Input: part model. Units: mm. Frame: model coordinates. Face numbers are marked on the shaded views. A direction names the side the tool comes from. Give positions to 0.01 mm unless a question says otherwise; leave off trailing zeros. Write each loop counter-clockwise with the first axis right and the second up, starting at its lowest first coordinate (ties: lowest second). Pieces come first, ordered by that corner, then holes.
```python
from build123d import *

# Parameters (mm, degrees)
SKETCH2_R           = 1.5
BOSS_EXTRUDE1_DEPTH = 2.5
SKETCH3_W           = 5.5
SKETCH3_H           = 2
BOSS_EXTRUDE2_DEPTH = 9
SKETCH4_W           = 5.5
SKETCH4_H           = 16.5
BOSS_EXTRUDE3_DEPTH = 2
SKETCH5_W           = 5.5
SKETCH5_H           = 2
BOSS_EXTRUDE4_DEPTH = 11.5
FILLET1_R           = 2


with BuildPart() as part:
    # Sketch2 → Boss-Extrude1 (new body)
    with BuildSketch(Plane(origin=(0, 0, 0), x_dir=(1, 0, 0), z_dir=(0, 1, 0))):
        with BuildLine():
            Line((-2.75, 0), (-2.75, 6.4))
            Line((-2.75, 6.4), (2.75, 6.4))
            Line((2.75, 6.4), (2.75, 0))
            ThreePointArc((2.75, 0), (0, -2.75), (-2.75, 0))
        make_face()
        with Locations(Location((0, 0, 0), (0, 0, 270))):
            Circle(SKETCH2_R, mode=Mode.SUBTRACT)
    extrude(amount=BOSS_EXTRUDE1_DEPTH)

    # Sketch3 → Boss-Extrude2 (add)
    with BuildSketch(Plane(origin=(0, 2.5, 0), x_dir=(1, 0, 0), z_dir=(0, 1, 0))):
        with Locations((0, 5.4)):
            Rectangle(SKETCH3_W, SKETCH3_H)
    extrude(amount=BOSS_EXTRUDE2_DEPTH)

    # Sketch4 → Boss-Extrude3 (add)
    with BuildSketch(Plane(origin=(0, 11.5, 0), x_dir=(1, 0, 0), z_dir=(0, 1, 0))):
        with Locations((0, 12.65)):
            Rectangle(SKETCH4_W, SKETCH4_H)
    extrude(amount=BOSS_EXTRUDE3_DEPTH)

    # Sketch5 → Boss-Extrude4 (add)
    with BuildSketch(Plane.XZ.offset(-11.5)):
        with Locations((0, -19.9)):
            Rectangle(SKETCH5_W, SKETCH5_H)
    extrude(amount=BOSS_EXTRUDE4_DEPTH)

    # Fillet1
    fillet1_edges = [part.edges().sort_by_distance(p)[0] for p in [
        (0, 13.5, -4.4),
        (0, 13.5, -20.9),
    ]]
    fillet(fillet1_edges, radius=FILLET1_R)


solid = part.part
```
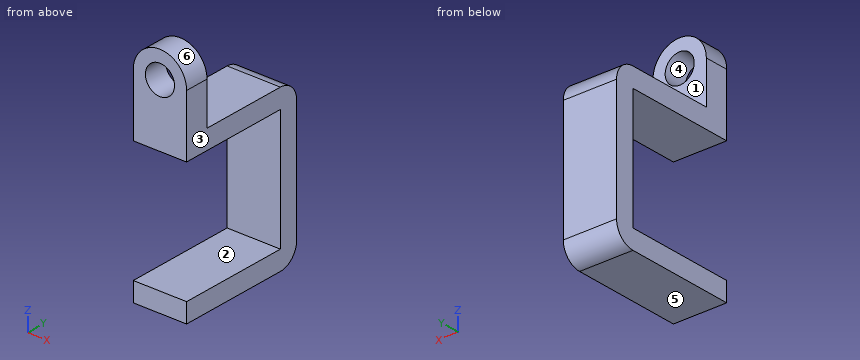
Item 1: Section B-B (x = 0). Return loops of the section in (y, z).
Item 2: Set-up query: the marked faces 1, 2 and 3. Return all of +Z, -Z, +X, -X, +Y, -Y with unobstructed straight access to the full face (end or side cutting, diameter ignored); none if empty.
Item 3: Ray query, line 1 (Z direction, x = 0.95, y = 7); line 2 (X direction, y = 1.2, z = 0); line 3 (Y direction, x = 2.2, z = -13). Return the intervals inside material, ascending.
Item 4: Pin query (flat end, axial travel): pin 1 (3 mm diameter, centred on x = 0, y = 5.5, fed in from +Z); pin 2 (5 mm diameter, centred on y = 2.5, z = -17.5, fed in from +X). Return the tip coordinate at first contact, or that it passes through.
Item 5: Section C-C (x = -2.05). Return loops of the section in (y, z), and give its area (3 significant figures).
Item 6: Section A-A (y = 4.5). Return loops of the section in (x, z).
Item 7: Mould query, pull axis X, two halves, no side actions, for the marked faces 4, 5 and 6. Classes: +X half, -X half, draft (parallel to the pull), parting line (faces both ways), or undercut.
Item 8: Section D-D (z = -2.5). Return loops of the section in (x, y).
Solved:
1. outline: (0, -20.9) - (11.5, -20.9) arc R2 ccw to (13.5, -18.9) - (13.5, -6.4) arc R2 ccw to (11.5, -4.4) - (2.5, -4.4) - (2.5, -1.5) - (0, -1.5) - (0, -6.4) - (11.5, -6.4) - (11.5, -18.9) - (0, -18.9) - close; (0, 1.5) - (2.5, 1.5) - (2.5, 2.75) - (0, 2.75) - close
2. face 1: +Z, +X, -X, +Y
2. face 2: +X, -X, -Y
2. face 3: +Z, -Z, +X, +Y, -Y
3. line 1: z = -20.9 to -18.9, -6.4 to -4.4
3. line 2: x = -2.75 to -1.5, 1.5 to 2.75
3. line 3: y = 11.5 to 13.5
4. pin 1: stops at z = -4.4
4. pin 2: stops at x = 2.75
5. outline: (0, -20.9) - (11.5, -20.9) arc R2 ccw to (13.5, -18.9) - (13.5, -6.4) arc R2 ccw to (11.5, -4.4) - (2.5, -4.4) - (2.5, 1.83) - (0, 1.83) - (0, -6.4) - (11.5, -6.4) - (11.5, -18.9) - (0, -18.9) - close
5. area: 92.9 mm2
6. outline: (-2.75, -20.9) - (2.75, -20.9) - (2.75, -18.9) - (-2.75, -18.9) - close; (-2.75, -6.4) - (2.75, -6.4) - (2.75, -4.4) - (-2.75, -4.4) - close
7. face 4: undercut
7. face 5: draft
7. face 6: parting line
8. outline: (-2.75, 0) - (2.75, 0) - (2.75, 2.5) - (-2.75, 2.5) - close
